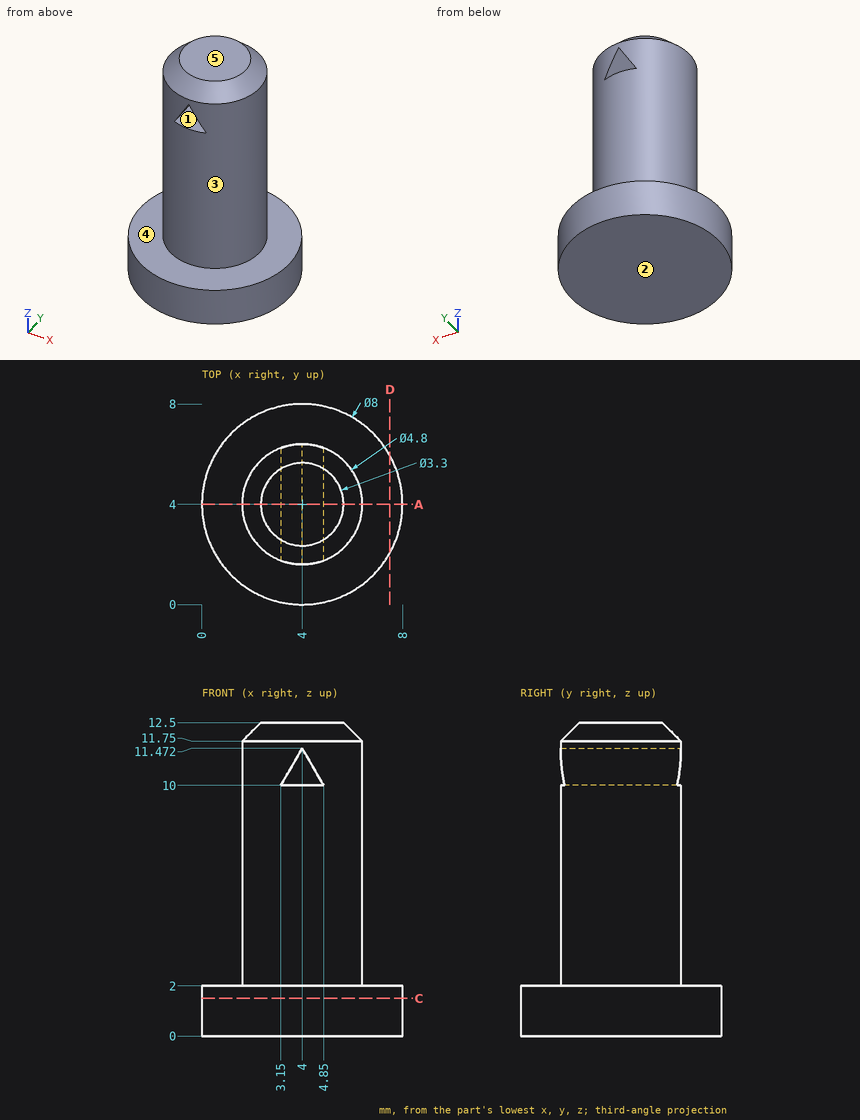
The figure shows three views and two pictorial views of one solid part (mm, origin at its lowest corner). Answer the questions. A direction names the side the tool comes from. Coordinates: 2 decimals unless noted, no trailing zeros. Loops run counter-clockwise (first coordinate to the right, second up) from the corner with the lowest first, then second, coordinate; pieces in that order, holes last. Notation, with made-up numbers: (-33, 74) -> (-28, 74) arc R18 cw to (-28, 87) -> close; hole circle Ø10 at (31, 56.25). An arc over 180 degrees is marked (long way). Return JSON: item names as keys, results as strings. Group by question number.
(1) A cutting plane is placed at C-C on z = 1.5. Write down the section's boundary in (x, y).
(2) Given pin 1 Ø3 at (x, z) = (7, 9.5) entering from +Y; pin 2 Ø2 at (y, z) = (1.5, 5.5) entering from +X, each flat-ended and moving along its own axis, determine where each tip first touches the part or whether it passes through.
(3) Determine the mould class of the marked faces 1, 2 and 3 for opening direction X: released by +X, released by -X, zero draft, split by the parting line, or undercut.
(4) Which of the six approach directions +Z, -Z, +X, -X, +Y, -Y give full straight-line access (tool end or side, diameter ignored) to the marked faces 4 and 5?
(5) A cutting plane is placed at D-D on x = 7.5. Write down the section's boundary in (y, z).
(6) A cutting plane is placed at A-A on y = 4. Write down the section's boundary in (x, z).
(7) Find the intervals of material crossed by probe 1 along Z at (x, y) = (7.5, 3); probe 2 along Z at (x, y) = (3.75, 4); probe 3 along Y at (x, z) = (3.75, 7), in increasing order. Write a range as from..to.
The answers:
{
 "1": {"outline": "circle Ø8 at (4, 4)"},
 "2": {"pin 1": "stops at y = 5.87", "pin 2": "stops at x = 5.87"},
 "3": {"face 1": "undercut", "face 2": "zero draft", "face 3": "split by the parting line"},
 "4": {"face 4": "+Z", "face 5": "+Z, +X, -X, +Y, -Y"},
 "5": {"outline": "(2.06, 0) -> (5.94, 0) -> (5.94, 2) -> (2.06, 2) -> close"},
 "6": {"outline": "(0, 0) -> (8, 0) -> (8, 2) -> (6.4, 2) -> (6.4, 11.75) -> (5.65, 12.5) -> (2.35, 12.5) -> (1.6, 11.75) -> (1.6, 2) -> (0, 2) -> close; hole (3.15, 10) -> (4.85, 10) -> (4, 11.47) -> close"},
 "7": {"probe 1": "z = 0..2", "probe 2": "z = 0..10, 11.04..12.5", "probe 3": "y = 1.61..6.39"}
}
